```python
from build123d import *

# Parameters (mm, degrees)
SKETCH1_R           = 2.675
SKETCH1_R_2         = 2.5
BOSS_EXTRUDE1_DEPTH = 3.5
FILLET1_R           = 3
SKETCH2_W           = 8.840351234
SKETCH2_H           = 3
SKETCH2_H_2         = 13
SKETCH2_R           = 2.5
SKETCH2_W_2         = 33.159648766
SKETCH2_R_2         = 4.125
SKETCH2_W_3         = 8.159648766
SKETCH2_H_3         = 4
BOSS_EXTRUDE2_DEPTH = 3.5
SKETCH2_4_W         = 8.840351234
SKETCH2_4_H         = 4
SKETCH2_4_H_2       = 13
SKETCH2_4_R         = 2.5
SKETCH2_4_H_3       = 3
SKETCH2_4_W_2       = 33.159648766
BOSS_EXTRUDE3_DEPTH = 24
FILLET2_R           = 3
SKETCH2_7_W         = 8.840351234
SKETCH2_7_H         = 3
BOSS_EXTRUDE5_DEPTH = 20.8
SKETCH2_9_R         = 2.5
CUT_EXTRUDE3_DEPTH  = 80.12322562
CUT_EXTRUDE1_DEPTH  = 80.12322562
SKETCH2_10_W        = 33.159648766
SKETCH2_10_H        = 3
SKETCH2_10_W_2      = 58.254565561
SKETCH2_10_H_2      = 4
BOSS_EXTRUDE6_DEPTH = 40
BOSS_EXTRUDE7_DEPTH = 15.25


with BuildPart() as part:
    # Sketch1 → Boss-Extrude1 (new body)
    with BuildSketch(Plane.XY):
        Polygon((-32.756938656, -9), (36.243061344, -9), (55.612607206, 13.908965344), (55.612607206, 50.908965344), (1.831518612, 50.908965344), align=None)
        with Locations((-17.168481388, 0)):
            Circle(SKETCH1_R, mode=Mode.SUBTRACT)
        with Locations((20.831518612, 0)):
            Circle(SKETCH1_R_2, mode=Mode.SUBTRACT)
        with Locations((1.831518612, 32.908965344)):
            Circle(SKETCH1_R_2, mode=Mode.SUBTRACT)
    extrude(amount=BOSS_EXTRUDE1_DEPTH)

    # Fillet1
    fillet1_edges = [part.edges().sort_by_distance(p)[0] for p in [
        (36.243061344, -9, 1.75),
        (-32.756938656, -9, 1.75),
        (1.831518612, 50.908965344, 1.75),
    ]]
    fillet(fillet1_edges, radius=FILLET1_R)

    # Sketch2 → Boss-Extrude2 (add)
    # profile 1 of 12: a face of its own
    with BuildSketch(Plane(origin=(0, 0, 0), x_dir=(-1, 0, 0), z_dir=(0, 0, -1))):
        with Locations((-50.751694229, 48.908965344)):
            Rectangle(SKETCH2_W, SKETCH2_H)
    # profile 2 of 12: a face of its own
    with BuildSketch(Plane(origin=(0, 0, 0), x_dir=(-1, 0, 0), z_dir=(0, 0, -1))):
        with Locations((-50.751694229, 40.908965344)):
            Rectangle(SKETCH2_W, SKETCH2_H_2)
        with Locations((-49.831518612, 40.908965344)):
            Circle(SKETCH2_R, mode=Mode.SUBTRACT)
    # profile 3 of 12: a face of its own
    with BuildSketch(Plane(origin=(0, 0, 0), x_dir=(-1, 0, 0), z_dir=(0, 0, -1))):
        with Locations((-29.751694229, 48.908965344)):
            Rectangle(SKETCH2_W_2, SKETCH2_H)
    # profile 4 of 12: a face of its own
    with BuildSketch(Plane(origin=(0, 0, 0), x_dir=(-1, 0, 0), z_dir=(0, 0, -1))):
        Polygon((-13.171869846, 47.408965344), (-46.331518612, 47.408965344), (-46.331518612, 34.408965344), (-46.331518612, 31.408965344), (-46.331518612, 18.408965344), (-13.171869846, 18.408965344), align=None)
    # profile 5 of 12: a face of its own
    with BuildSketch(Plane(origin=(0, 0, 0), x_dir=(-1, 0, 0), z_dir=(0, 0, -1))):
        with Locations((-50.751694229, 32.908965344)):
            Rectangle(SKETCH2_W, SKETCH2_H)
    # profile 6 of 12: a face of its own
    with BuildSketch(Plane(origin=(0, 0, 0), x_dir=(-1, 0, 0), z_dir=(0, 0, -1))):
        Polygon((12.168481388, 47.408965344), (-13.171869846, 47.408965344), (-13.171869846, 18.408965344), (11.923046949, 18.408965344), (12.168481388, 18.408965344), (12.168481388, 31.408965344), (12.168481388, 34.408965344), align=None)
        with Locations((-1.831518612, 32.908965344)):
            Circle(SKETCH2_R_2, mode=Mode.SUBTRACT)
    # profile 7 of 12: a face of its own
    with BuildSketch(Plane(origin=(0, 0, 0), x_dir=(-1, 0, 0), z_dir=(0, 0, -1))):
        with Locations((-50.751694229, 24.908965344)):
            Rectangle(SKETCH2_W, SKETCH2_H_2)
        with Locations((-49.831518612, 24.908965344)):
            Circle(SKETCH2_R, mode=Mode.SUBTRACT)
    # profile 8 of 12: a face of its own
    with BuildSketch(Plane(origin=(0, 0, 0), x_dir=(-1, 0, 0), z_dir=(0, 0, -1))):
        with Locations((16.248305771, 40.908965344)):
            Rectangle(SKETCH2_W_3, SKETCH2_H_2)
        with Locations((16.168481388, 40.908965344)):
            Circle(SKETCH2_R, mode=Mode.SUBTRACT)
    # profile 9 of 12: a face of its own
    with BuildSketch(Plane(origin=(0, 0, 0), x_dir=(-1, 0, 0), z_dir=(0, 0, -1))):
        Polygon((11.923046949, 18.408965344), (-13.171869846, 18.408965344), (-46.331518612, 18.408965344), (-46.331518612, 14.408965344), (11.923046949, 14.408965344), align=None)
    # profile 10 of 12: a face of its own
    with BuildSketch(Plane(origin=(0, 0, 0), x_dir=(-1, 0, 0), z_dir=(0, 0, -1))):
        with Locations((-50.751694229, 16.408965344)):
            Rectangle(SKETCH2_W, SKETCH2_H_3)
    # profile 11 of 12: a face of its own
    with BuildSketch(Plane(origin=(0, 0, 0), x_dir=(-1, 0, 0), z_dir=(0, 0, -1))):
        with Locations((16.248305771, 32.908965344)):
            Rectangle(SKETCH2_W_3, SKETCH2_H)
    # profile 12 of 12: a face of its own
    with BuildSketch(Plane(origin=(0, 0, 0), x_dir=(-1, 0, 0), z_dir=(0, 0, -1))):
        Polygon((20.328130154, 31.408965344), (12.168481388, 31.408965344), (12.168481388, 18.408965344), (16.168481388, 18.408965344), (20.328130154, 18.408965344), align=None)
        with Locations((16.168481388, 24.908965344)):
            Circle(SKETCH2_R, mode=Mode.SUBTRACT)
    extrude(amount=-BOSS_EXTRUDE2_DEPTH)

    # Sketch2<4> → Boss-Extrude3 (add)
    # profile 1 of 6: a face of its own
    with BuildSketch(Plane(origin=(0, 0, 0), x_dir=(-1, 0, 0), z_dir=(0, 0, -1))):
        Polygon((11.923046949, 18.408965344), (-13.171869846, 18.408965344), (-46.331518612, 18.408965344), (-46.331518612, 14.408965344), (11.923046949, 14.408965344), align=None)
    # profile 2 of 6: a face of its own
    with BuildSketch(Plane(origin=(0, 0, 0), x_dir=(-1, 0, 0), z_dir=(0, 0, -1))):
        with Locations((-50.751694229, 16.408965344)):
            Rectangle(SKETCH2_4_W, SKETCH2_4_H)
    # profile 3 of 6: a face of its own
    with BuildSketch(Plane(origin=(0, 0, 0), x_dir=(-1, 0, 0), z_dir=(0, 0, -1))):
        with Locations((-50.751694229, 24.908965344)):
            Rectangle(SKETCH2_4_W, SKETCH2_4_H_2)
        with Locations((-49.831518612, 24.908965344)):
            Circle(SKETCH2_4_R, mode=Mode.SUBTRACT)
    # profile 4 of 6: a face of its own
    with BuildSketch(Plane(origin=(0, 0, 0), x_dir=(-1, 0, 0), z_dir=(0, 0, -1))):
        with Locations((-50.751694229, 40.908965344)):
            Rectangle(SKETCH2_4_W, SKETCH2_4_H_2)
        with Locations((-49.831518612, 40.908965344)):
            Circle(SKETCH2_4_R, mode=Mode.SUBTRACT)
    # profile 5 of 6: a face of its own
    with BuildSketch(Plane(origin=(0, 0, 0), x_dir=(-1, 0, 0), z_dir=(0, 0, -1))):
        with Locations((-50.751694229, 48.908965344)):
            Rectangle(SKETCH2_4_W, SKETCH2_4_H_3)
    # profile 6 of 6: a face of its own
    with BuildSketch(Plane(origin=(0, 0, 0), x_dir=(-1, 0, 0), z_dir=(0, 0, -1))):
        with Locations((-29.751694229, 48.908965344)):
            Rectangle(SKETCH2_4_W_2, SKETCH2_4_H_3)
    extrude(amount=BOSS_EXTRUDE3_DEPTH)

    # Fillet2
    # the kernel refuses this fillet: 3 mm, written as the material it adds along each edge
    with BuildSketch(Plane(origin=(-16.932365136, 18.408965344, 3.5), x_dir=(-0.49999999999999933, -0.8660254037844389, 0), z_dir=(0, 0, -1))) as fillet2_piece_1:
        with BuildLine():
            CenterArc((4.697298716, 3), FILLET2_R, 181.130351539, 88.869648461)
            Line((1.697882509, 2.940818771), (1.637894185, 2.939635146))
            ThreePointArc((1.637894185, 2.939635146), (0.79697973, 1.500409385), (-0.051961524, 0.03))
            Line((-0.051961524, 0.03), (0, -0.06))
            Line((0, -0.06), (4.697298716, -0.06))
            Line((4.697298716, -0.06), (4.697298716, 0))
        make_face()
    extrude(amount=3.5)

    # Sketch2<7> → Boss-Extrude5 (add)
    with BuildSketch(Plane(origin=(0, 0, 0), x_dir=(-1, 0, 0), z_dir=(0, 0, -1))):
        with Locations((-50.751694229, 32.908965344)):
            Rectangle(SKETCH2_7_W, SKETCH2_7_H)
    extrude(amount=BOSS_EXTRUDE5_DEPTH)

    # Sketch2<9> → Cut-Extrude3 (cut, through all)
    with BuildSketch(Plane(origin=(0, 0, 0), x_dir=(-1, 0, 0), z_dir=(0, 0, -1))):
        with Locations((-49.831518612, 40.908965344)):
            Circle(SKETCH2_9_R)
        with Locations((-49.831518612, 24.908965344)):
            Circle(SKETCH2_9_R)
    extrude(amount=-CUT_EXTRUDE3_DEPTH, mode=Mode.SUBTRACT)

    # Sketch3 → Cut-Extrude1 (cut, through all)
    with BuildSketch(Plane(origin=(0, 0, 0), x_dir=(-1, 0, 0), z_dir=(0, 0, -1))):
        Polygon((-1.831518612, 50.908965344), (32.756938656, -9), (32.756938656, 50.908965344), align=None)
    extrude(amount=-CUT_EXTRUDE1_DEPTH, mode=Mode.SUBTRACT)

    # Sketch2<10> → Boss-Extrude6 (add)
    with BuildSketch(Plane(origin=(0, 0, 0), x_dir=(-1, 0, 0), z_dir=(0, 0, -1))):
        with Locations((-29.751694229, 48.908965344)):
            Rectangle(SKETCH2_10_W, SKETCH2_10_H)
        with Locations((-17.204235832, 16.408965344)):
            Rectangle(SKETCH2_10_W_2, SKETCH2_10_H_2)
    extrude(amount=BOSS_EXTRUDE6_DEPTH)

    # Sketch2<11> → Boss-Extrude7 (add)
    with BuildSketch(Plane(origin=(0, 0, 0), x_dir=(-1, 0, 0), z_dir=(0, 0, -1))):
        Polygon((-13.171869846, 47.408965344), (-46.331518612, 47.408965344), (-46.331518612, 34.408965344), (-46.331518612, 31.408965344), (-46.331518612, 18.408965344), (-13.171869846, 18.408965344), align=None)
    extrude(amount=BOSS_EXTRUDE7_DEPTH)


solid = part.part
```
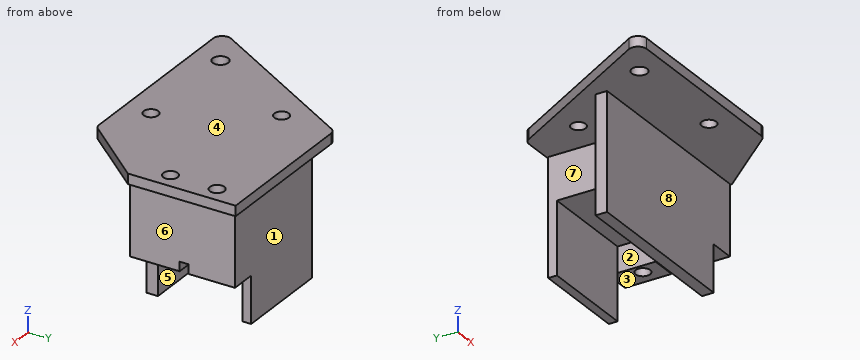
Build history of the part. All positions in model axes, mm. Face numbers are marked on the shaded views. A direction names the side the tool comes from. Round coordinates to 2 decimals unless told otherwise and drop trailing zeros. Order: outer loops, then holes, each group sorted by start corner. A loop starts at its lowest first (then second) coordinate and runs counter-clockwise, first axis right, second up. Notation, with made-up numbers: (-31.75, 46) -> (22.25, 46) arc R7 cw to (22.25, 53) -> close; hole circle Ø8 at (-22, -2.5). An arc over 180 degrees is marked (long way). Answer in a Markdown table with one row per item.
1) Band-saw the part on D-D on y = 0. Give the cut face in (x, z), and give its area (3 significant figures).
Values:
| item | result |
|---|---|
| outline | (-27.56, 0) -> (-19.84, 0) -> (-19.84, 3.5) -> (-27.56, 3.5) -> close; (-14.49, 0) -> (18.33, 0) -> (18.33, 3.5) -> (-14.49, 3.5) -> close; (23.33, 0) -> (43.85, 0) -> (43.85, 3.5) -> (23.33, 3.5) -> close |
| area | 214 mm2 |
2) Band-saw the part on B-B on x = 30.5. Give the cut face in (y, z).
Values:
| item | result |
|---|---|
| outline | (-9, 0) -> (14.41, 0) -> (14.41, -40) -> (18.41, -40) -> (18.41, -15.25) -> (47.41, -15.25) -> (47.41, -40) -> (50.41, -40) -> (50.41, 0) -> (50.91, 0) -> (50.91, 3.5) -> (-9, 3.5) -> close |
3) Wall check: L1, parallel to Y at x = 44, z = -24.5; L2, parallel to Y at x = 20.5, z = -1; L3, parallel to Z at x = 28.5, y = 21. Give the ranges that are in metal, low to high.
Values:
| item | result |
|---|---|
| L1 | 14.41 to 18.41, 47.41 to 50.41 |
| L2 | 14.41 to 50.41 |
| L3 | -15.25 to 3.5 |
4) Band-saw the part on A-A on z = -26.5. Give the cut face in (x, y), and give its area (3 significant figures).
Values:
| item | result |
|---|---|
| outline | (-11.92, 14.41) -> (46.33, 14.41) -> (46.33, 18.41) -> (-11.92, 18.41) -> close; (13.17, 47.41) -> (46.33, 47.41) -> (46.33, 50.41) -> (13.17, 50.41) -> close |
| area | 332 mm2 |
5) Mould opens along Y. For the marked faces 1, 2 and 3 say: released by +Y, released by -Y, zero draft, split by the parting line, or undercut.
Values:
| item | result |
|---|---|
| face 1 | released by +Y |
| face 2 | undercut |
| face 3 | zero draft |
6) Which spindle directions (+Z, -Z, +X, -X, +Y, -Y) get a long thin tool onto all of the face, cutting with end or side? Do the marked faces 4, 5, 6, 7 and 8. Say none if no direction does.
Values:
| item | result |
|---|---|
| face 4 | +Z, +X, -X, +Y, -Y |
| face 5 | -Z, -X |
| face 6 | -Z, +X, +Y, -Y |
| face 7 | -Z, -X, +Y |
| face 8 | -Z, +X, -X, -Y |
7) Pin check, flat tips, straight feed: P1, Ø12, axis at x = 9.5, y = 4, coming from the -Z side; P2, Ø6, axis at x = -10, z = -12.5, coming from the +Y side; P3, Ø2.5, axis at y = 27, z = -18.5, coming from the -X side; P4, Ø2, axis at x = -13.5, z = -25.5, coming from the -Y side. Stop position of each tip, or through.
Values:
| item | result |
|---|---|
| P1 | z = 0 |
| P2 | y = 18.41 |
| P3 | x = 46.33 |
| P4 | through |
8) Band-saw the part on C-C on y = 26.5. Give the cut face in (x, z), and give its area (3 significant figures).
Values:
| item | result |
|---|---|
| outline | (-12.26, 0) -> (13.17, 0) -> (13.17, -15.25) -> (46.33, -15.25) -> (46.33, -24) -> (47.9, -24) -> (47.9, 3.5) -> (-12.26, 3.5) -> close; (51.76, -24) -> (55.17, -24) -> (55.17, 0) -> (55.61, 0) -> (55.61, 3.5) -> (51.76, 3.5) -> close |
| area | 849 mm2 |
